from build123d import *

# Parameters (mm, degrees)
BOSS_EXTRUDE1_DEPTH                      = 1.5
MIRROR1_AT_THE_SECOND_PLANE_COPY_1_DEPTH = 1.5
SCALE1_SCALE                             = 0.5


with BuildPart() as part:
    # Sketch1 → Boss-Extrude1 (new, symmetric)
    with BuildSketch(Plane(origin=(0, 0, 0), x_dir=(1, 0, 0), z_dir=(0, 1, 0))):
        with BuildLine():
            Line((0, 3), (16.5, 3))
            ThreePointArc((16.5, 3), (21.385877083, 3.880236087), (25.657364834, 6.41025641))
            ThreePointArc((25.657364834, 6.41025641), (33.285021532, 10.928149844), (42.009802038, 12.5))
            Line((42.009802038, 12.5), (57.5, 12.5))
            Line((57.5, 12.5), (57.5, 0))
            Line((57.5, 0), (0, 0))
            Line((0, 0), (0, 3))
        make_face()
    boss_extrude1 = extrude(amount=BOSS_EXTRUDE1_DEPTH, both=True)



with BuildPart() as mirror1_1:
    # Mirror1: Boss-Extrude1 across plane
    add(boss_extrude1.mirror(Plane(origin=(0, 0, 0), x_dir=(0, 0, 1), z_dir=(1, 0, 0))))


with BuildPart() as part_1:
    add(part.part)

    add(mirror1_1.part)  # Mirror1 at the second plane merges Mirror1_1
    # Mirror1 at the second plane: Boss-Extrude1 across plane
    add(boss_extrude1.mirror(Plane.XY))

    # Mirror1 at the second plane copy 1 sketc → Mirror1 at the second plane copy 1 (add, symmetric)
    with BuildSketch(Plane(origin=(0, 0, 0), x_dir=(-1, 0, 0), z_dir=(0, 1, 0))):
        with BuildLine():
            Line((0, 3), (16.5, 3))
            ThreePointArc((16.5, 3), (21.385877083, 3.880236087), (25.657364834, 6.41025641))
            ThreePointArc((25.657364834, 6.41025641), (33.285021532, 10.928149844), (42.009802038, 12.5))
            Line((42.009802038, 12.5), (57.5, 12.5))
            Line((57.5, 12.5), (57.5, 0))
            Line((57.5, 0), (0, 0))
            Line((0, 0), (0, 3))
        make_face()
    extrude(amount=MIRROR1_AT_THE_SECOND_PLANE_COPY_1_DEPTH, both=True)


with BuildPart() as part_2:
    # Scale1: scaled about (0, 0, 0)
    add(part_1.part.scale(SCALE1_SCALE))


solid = part_2.part
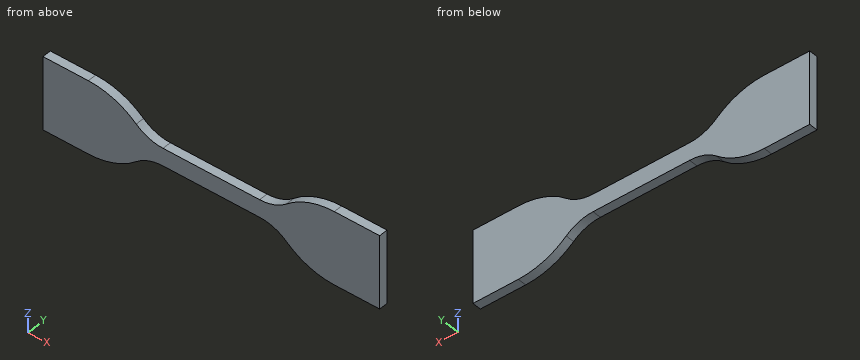
The listing builds one solid part. Answer for the finished solid, in the listing's coordinates (mm). Give positions to 0.01 mm unless a question says otherwise; leave off trailing zeros. Order: outer loops, then holes, each group sorted by start corner. A loop starts at its lowest first (then second) coordinate and runs counter-clockwise, first axis right, second up. Notation, with made-up numbers: (24, -31.5) - (54, -31.5) arc R23 cw to (54, -3.5) - close; hole circle Ø9 at (-27, 42). An arc over 180 degrees is marked (long way). Answer as CSV lines item,"result".
Q1. A cutting plane is placed at B-B, the plane y = -0.45. Determine the outline of the cut face in (x, z).
Answer key:
outline,"(-28.75, -6.25) - (-21, -6.25) arc R12.5 ccw to (-12.83, -3.21) arc R7 cw to (-8.25, -1.5) - (8.25, -1.5) arc R7 cw to (12.83, -3.21) arc R12.5 ccw to (21, -6.25) - (28.75, -6.25) - (28.75, 6.25) - (21, 6.25) arc R12.5 ccw to (12.83, 3.21) arc R7 cw to (8.25, 1.5) - (-8.25, 1.5) arc R7 cw to (-12.83, 3.21) arc R12.5 ccw to (-21, 6.25) - (-28.75, 6.25) - close"
Q2. A cutting plane is placed at C-C, the plane x = 7. Determine the outline of the cut face in (y, z).
Answer key:
outline,"(-0.75, -1.5) - (0.75, -1.5) - (0.75, 1.5) - (-0.75, 1.5) - close"
Q3. Straight lines are drawn through the part: L1, parallel to X at y = -0.15, z = 2.25; L2, parallel to X at y = -0.35, z = -3; L3, parallel to Z at x = -5.5, y = 0.05. For each, find the intervals that lie inside material, in ascending order.
Answer key:
L1,"x = -28.75 to -11.4, 11.4 to 28.75"
L2,"x = -28.75 to -12.58, 12.58 to 28.75"
L3,"z = -1.5 to 1.5"
Q4. A cutting plane is placed at A-A, the plane z = -4.5. Determine the outline of the cut face in (x, y), and give its area (3 significant figures).
Answer key:
outline,"(-28.75, -0.75) - (-14.63, -0.75) - (-14.63, 0.75) - (-28.75, 0.75) - close; (14.63, -0.75) - (28.75, -0.75) - (28.75, 0.75) - (14.63, 0.75) - close"
area,"42.4 mm^2"
Q5. A cutting plane is placed at D-D, the plane z = 5.25. Determine the outline of the cut face in (x, y).
Answer key:
outline,"(-28.75, -0.75) - (-16.11, -0.75) - (-16.11, 0.75) - (-28.75, 0.75) - close; (16.11, -0.75) - (28.75, -0.75) - (28.75, 0.75) - (16.11, 0.75) - close"
